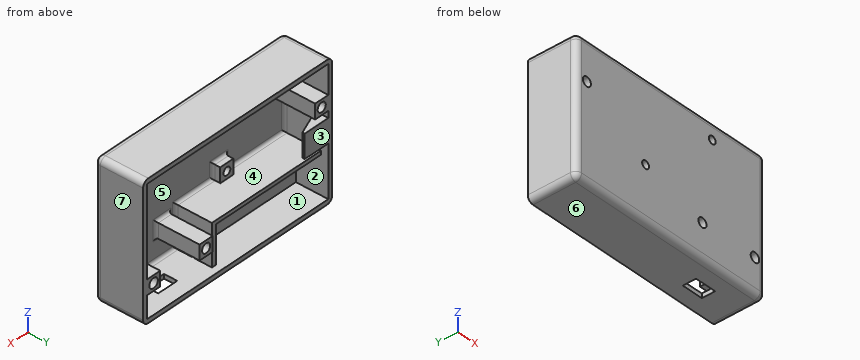
```python
from build123d import *

# Parameters (mm, degrees)
CROQUIS1_W               = 138
CROQUIS1_H               = 85
SALIENTE_EXTRUIR1_DEPTH  = 3
CROQUIS3_W               = 144
CROQUIS3_H               = 91
CROQUIS3_W_2             = 138
CROQUIS3_H_2             = 85
SALIENTE_EXTRUIR3_DEPTH  = 3
CROQUIS7_W               = 144
CROQUIS7_H               = 91
CROQUIS7_W_2             = 138
CROQUIS7_H_2             = 85
SALIENTE_EXTRUIR4_DEPTH  = 30
CROQUIS8_W               = 10
CROQUIS8_H               = 10
SALIENTE_EXTRUIR5_DEPTH  = 5.5
CROQUIS9_W               = 16
CROQUIS9_H               = 1.5
SALIENTE_EXTRUIR6_DEPTH  = 18
SALIENTE_EXTRUIR7_DEPTH  = 16
CROQUIS11_W              = 83
CROQUIS11_H              = 28
SALIENTE_EXTRUIR8_DEPTH  = 8
SALIENTE_EXTRUIR9_DEPTH  = 17
CORTAR_EXTRUIR1_REACH    = 102.241
CROQUIS14_R              = 2.5
CORTAR_EXTRUIR2_REACH    = 90.626
CROQUIS15_R              = 2.6
CORTAR_EXTRUIR3_REACH    = 120.393
CROQUIS16_W              = 14.5
CROQUIS16_H              = 9
CROQUIS17_W              = 10
CROQUIS17_H              = 10
SALIENTE_EXTRUIR10_DEPTH = 30
CORTAR_EXTRUIR4_REACH    = 93.341
CROQUIS18_R              = 3.1
CROQUIS18_R_2            = 3.25
REDONDEO1_R              = 2
REDONDEO2_R              = 4
CORTAR_EXTRUIR5_REACH    = 90.626
CROQUIS21_R              = 2.6


with BuildPart() as part:
    # Croquis1 → Saliente-Extruir1 (new body)
    with BuildSketch(Plane(origin=(0, 0, 0), x_dir=(1, 0, 0), z_dir=(0, 1, 0))):
        Rectangle(CROQUIS1_W, CROQUIS1_H)
    extrude(amount=SALIENTE_EXTRUIR1_DEPTH)

    # Croquis3 → Saliente-Extruir3 (add)
    with BuildSketch(Plane(origin=(0, 3, 0), x_dir=(1, 0, 0), z_dir=(0, 1, 0))):
        Rectangle(CROQUIS3_W, CROQUIS3_H)
        Rectangle(CROQUIS3_W_2, CROQUIS3_H_2, mode=Mode.SUBTRACT)
    extrude(amount=-SALIENTE_EXTRUIR3_DEPTH)

    # Croquis7 → Saliente-Extruir4 (add)
    with BuildSketch(Plane(origin=(0, 3, 0), x_dir=(1, 0, 0), z_dir=(0, 1, 0))):
        Rectangle(CROQUIS7_W, CROQUIS7_H)
        Rectangle(CROQUIS7_W_2, CROQUIS7_H_2, mode=Mode.SUBTRACT)
    extrude(amount=SALIENTE_EXTRUIR4_DEPTH)

    # Croquis8 → Saliente-Extruir5 (add)
    with BuildSketch(Plane(origin=(0, 3, 0), x_dir=(1, 0, 0), z_dir=(0, 1, 0))):
        with Locations((-19.2, 9.5)):
            Rectangle(CROQUIS8_W, CROQUIS8_H)
        with Locations((31.5, -33.5)):
            Rectangle(CROQUIS8_W, CROQUIS8_H)
    extrude(amount=SALIENTE_EXTRUIR5_DEPTH)

    # Croquis9 → Saliente-Extruir6 (add)
    with BuildSketch(Plane(origin=(-69, 0, 0), x_dir=(0, 0, -1), z_dir=(1, 0, 0))):
        with Locations((-0.5, 32.25)):
            Rectangle(CROQUIS9_W, CROQUIS9_H)
    extrude(amount=SALIENTE_EXTRUIR6_DEPTH)

    # Croquis10 → Saliente-Extruir7 (add)
    with BuildSketch(Plane.XY.offset(8.5)):
        Polygon((-51, 31.5), (-69, 24.227527935), (-69, 33), (-51, 33), align=None)
    extrude(amount=-SALIENTE_EXTRUIR7_DEPTH)

    # Croquis11 → Saliente-Extruir8 (add)
    with BuildSketch(Plane(origin=(0, 3, 0), x_dir=(1, 0, 0), z_dir=(0, 1, 0))):
        with Locations((-27.5, 28.5)):
            Rectangle(CROQUIS11_W, CROQUIS11_H)
    extrude(amount=SALIENTE_EXTRUIR8_DEPTH)

    # Croquis12 → Saliente-Extruir9 (add)
    with BuildSketch(Plane(origin=(0, 11, 0), x_dir=(1, 0, 0), z_dir=(0, 1, 0))):
        Polygon((14, 42.5), (11, 42.5), (11, 17), (-69, 17), (-69, 14.5), (14, 14.5), align=None)
    extrude(amount=SALIENTE_EXTRUIR9_DEPTH)

    # Croquis14 → Cortar-Extruir1 (cut, up to next)
    with BuildSketch(Plane.ZY.offset(-11), mode=Mode.PRIVATE) as cortar_extruir1_sk1:
        with Locations(Location((-40, 15.5, 0), (0, 0, 180))):
            Circle(CROQUIS14_R)
    cortar_extruir1_tool1 = extrude(cortar_extruir1_sk1.sketch, amount=-CORTAR_EXTRUIR1_REACH, mode=Mode.PRIVATE) & part.part
    add(cortar_extruir1_tool1.solids().sort_by_distance((11, 15.5, -40))[0], mode=Mode.SUBTRACT)

    # Croquis15 → Cortar-Extruir2 (cut, up to next)
    with BuildSketch(Plane(origin=(0, 8.5, 0), x_dir=(1, 0, 0), z_dir=(0, 1, 0)), mode=Mode.PRIVATE) as cortar_extruir2_sk1:
        with Locations(Location((31.5, -33.5, 0), (0, 0, 270))):
            Circle(CROQUIS15_R)
    cortar_extruir2_tool1 = extrude(cortar_extruir2_sk1.sketch, amount=-CORTAR_EXTRUIR2_REACH, mode=Mode.PRIVATE) & part.part
    add(cortar_extruir2_tool1.solids().sort_by_distance((31.5, 8.5, 33.5))[0], mode=Mode.SUBTRACT)

    # Croquis16 → Cortar-Extruir3 (cut, up to next)
    with BuildSketch(Plane.XY.offset(-42.5), mode=Mode.PRIVATE) as cortar_extruir3_sk1:
        with Locations((41.5, 18)):
            Rectangle(CROQUIS16_W, CROQUIS16_H)
    cortar_extruir3_tool1 = extrude(cortar_extruir3_sk1.sketch, amount=-CORTAR_EXTRUIR3_REACH, mode=Mode.PRIVATE) & part.part
    add(cortar_extruir3_tool1.solids().sort_by_distance((41.5, 18, -42.5))[0], mode=Mode.SUBTRACT)

    # Croquis17 → Saliente-Extruir10 (add)
    with BuildSketch(Plane(origin=(0, 3, 0), x_dir=(1, 0, 0), z_dir=(0, 1, 0))):
        with Locations((-64, -18)):
            Rectangle(CROQUIS17_W, CROQUIS17_H)
        with Locations((64, 22.5)):
            Rectangle(CROQUIS17_W, CROQUIS17_H)
        with Locations((24, 22.5)):
            Rectangle(CROQUIS17_W, CROQUIS17_H)
    extrude(amount=SALIENTE_EXTRUIR10_DEPTH)

    # Croquis18 → Cortar-Extruir4 (cut, up to next)
    with BuildSketch(Plane(origin=(0, 33, 0), x_dir=(1, 0, 0), z_dir=(0, 1, 0)), mode=Mode.PRIVATE) as cortar_extruir4_sk1:
        with Locations(Location((-64, -18, 0), (0, 0, 270))):
            Circle(CROQUIS18_R)
    cortar_extruir4_tool1 = extrude(cortar_extruir4_sk1.sketch, amount=-CORTAR_EXTRUIR4_REACH, mode=Mode.PRIVATE) & part.part
    # Croquis18 → Cortar-Extruir4 (cut, up to next)
    with BuildSketch(Plane(origin=(0, 33, 0), x_dir=(1, 0, 0), z_dir=(0, 1, 0)), mode=Mode.PRIVATE) as cortar_extruir4_sk2:
        with Locations(Location((24, 22.5, 0), (0, 0, 270))):
            Circle(CROQUIS18_R)
    cortar_extruir4_tool2 = extrude(cortar_extruir4_sk2.sketch, amount=-CORTAR_EXTRUIR4_REACH, mode=Mode.PRIVATE) & part.part
    # Croquis18 → Cortar-Extruir4 (cut, up to next)
    with BuildSketch(Plane(origin=(0, 33, 0), x_dir=(1, 0, 0), z_dir=(0, 1, 0)), mode=Mode.PRIVATE) as cortar_extruir4_sk3:
        with Locations(Location((64, 22.5, 0), (0, 0, 270))):
            Circle(CROQUIS18_R_2)
    cortar_extruir4_tool3 = extrude(cortar_extruir4_sk3.sketch, amount=-CORTAR_EXTRUIR4_REACH, mode=Mode.PRIVATE) & part.part
    add(cortar_extruir4_tool1.solids().sort_by_distance((-64, 33, 18))[0], mode=Mode.SUBTRACT)
    add(cortar_extruir4_tool2.solids().sort_by_distance((24, 33, -22.5))[0], mode=Mode.SUBTRACT)
    add(cortar_extruir4_tool3.solids().sort_by_distance((64, 33, -22.5))[0], mode=Mode.SUBTRACT)

    # Redondeo1
    redondeo1_edges = [part.edges().sort_by_distance(p)[0] for p in [
        (-69, 3, -0.75),
        (-0.1, 3, -14.5),
        (-46.6, 3, -14.5),
        (14, 3, -28.5),
        (-69, 3, 32.75),
        (-64, 3, 23),
        (-59, 3, 18),
        (-64, 3, 13),
        (69, 3, -35),
        (64, 3, -27.5),
        (59, 3, -22.5),
        (64, 3, -17.5),
        (19, 3, -22.5),
        (24, 3, -17.5),
        (29, 3, -22.5),
        (24, 3, -27.5),
        (0, 3, 42.5),
        (69, 3, 12.5),
        (41.5, 3, -42.5),
        (-14.2, 3, -9.5),
        (-24.2, 3, -9.5),
        (-19.2, 3, -4.5),
        (36.5, 3, 33.5),
        (31.5, 3, 28.5),
        (26.5, 3, 33.5),
        (31.5, 3, 38.5),
    ]]
    fillet(redondeo1_edges, radius=REDONDEO1_R - 0.0001)  # a hair under: the kernel refuses the full size

    # Redondeo2
    redondeo2_edges = [part.edges().sort_by_distance(p)[0] for p in [
        (0, 0, 45.5),
        (72, 16.5, 45.5),
        (-72, 0, 0),
        (-72, 16.5, 45.5),
        (0, 0, -45.5),
        (-72, 16.5, -45.5),
        (72, 0, 0),
        (72, 16.5, -45.5),
    ]]
    fillet(redondeo2_edges, radius=REDONDEO2_R)

    # Croquis21 → Cortar-Extruir5 (cut, up to next)
    with BuildSketch(Plane(origin=(0, 8.5, 0), x_dir=(1, 0, 0), z_dir=(0, 1, 0)), mode=Mode.PRIVATE) as cortar_extruir5_sk1:
        with Locations(Location((-19.3, 9.7, 0), (0, 0, 270))):
            Circle(CROQUIS21_R)
    cortar_extruir5_tool1 = extrude(cortar_extruir5_sk1.sketch, amount=-CORTAR_EXTRUIR5_REACH, mode=Mode.PRIVATE) & part.part
    add(cortar_extruir5_tool1.solids().sort_by_distance((-19.3, 8.5, -9.7))[0], mode=Mode.SUBTRACT)


solid = part.part
```
The listing builds one solid part. Answer for the finished solid, in the listing's coordinates (mm). Face numbers are marked on the shaded views. A direction names the side the tool comes from. Round coordinates to 2 decimals unless told otherwise and drop trailing zeros. Loops run counter-clockwise (first coordinate to the right, second up) from the corner with the lowest first, then second, coordinate; pieces in that order, holes last. Notation, with made-up numbers: (41, 52.5) - (93, 52.5) arc R16 ccw to (93, 58.5) - close; hole circle Ø2 at (5.5, -27). An arc over 180 degrees is marked (long way). Use one line per item in the form item = value. Start each with the question number.
1. For a pull along Z with two mould halves and no side action, classify the marked faces 4, 5, 6 and 7 as pulls with the +Z half, pulls with the -Z half, needs draft (parallel to the pull), parting line crosses it, or undercut.
2. The part is cut by section B-B on y = 29.5. Give the number of separate pieces and of enclosed holes in the cut face, then the cut area to 3 significant figures.
3. The part is cut by section D-D on x = -35. Determine the outline of the cut face in (y, z), then the cut area to 3 significant figures.
4. Consider line 1 (Z direction, x = 8, y = 18.5); line 2 (X direction, y = 10, z = -22.5); line 3 (X direction, y = 18, z = -33.5). Determine where each line is inside the solid, lowest interval first. Write a range as [from, to].
5. Given pin 1 Ø7.5 at (x, z) = (-27.5, -28) entering from +Y; pin 2 Ø4 at (x, z) = (31.5, 33.5) entering from -Y, each flat-ended and moving along its own axis, determine where each tip first touches the part or whether it passes through.
6. A tool of negligible diameter and unlimited length cuts with its end or side. For the marked faces 1, 2 and 3, from which of +Z, -Z, +X, -X, +Y, -Y can it reach the whole face along a straight path? Write none if from no direction.
7. The part is cut by section A-A on z = 18. Determine the outline of the cut face in (x, y), then the cut area to 3 significant figures.
Geometry check:
q1.face_4 = undercut
q1.face_5 = undercut
q1.face_6 = pulls with the -Z half
q1.face_7 = needs draft
q2.separate_pieces = 2
q2.enclosed_holes = 4
q2.area = 1,780 mm^2
q3.outline = (0, -41.5) arc R4 ccw to (4, -45.5) - (33, -45.5) - (33, -42.5) - (11, -42.5) - (11, -17) - (28, -17) - (28, -14.5) - (5, -14.5) arc R2 cw to (3, -12.5) - (3, 40.5) arc R2 cw to (5, 42.5) - (33, 42.5) - (33, 45.5) - (4, 45.5) arc R4 ccw to (0, 41.5) - close
q3.area = 714 mm^2
q4.line_1 = [-45.5, -42.5], [-17, -14.5], [42.5, 45.5]
q4.line_2 = [-72, 14], [19, 20.9], [27.1, 29], [59, 60.75], [67.25, 72]
q4.line_3 = [-72, -69], [11, 14], [69, 72]
q5.pin_1 = 11
q5.pin_2 = through
q6.face_1 = +Y
q6.face_2 = none
q6.face_3 = +Z, -Z, +X, -X, +Y
q7.outline = (-72, 4) arc R4 ccw to (-68, 0) - (-67.1, 0) - (-67.1, 33) - (-72, 33) - close; (-60.9, 0) - (68, 0) arc R4 ccw to (72, 4) - (72, 33) - (69, 33) - (69, 5) arc R2 cw to (67, 3) - (-57, 3) arc R2 cw to (-59, 5) - (-59, 33) - (-60.9, 33) - close
q7.area = 702 mm^2
